Build history of the part. All positions in model axes, mm. A direction names the side the tool comes from. Give positions to 0.01 mm unless a question says otherwise; leave off trailing zeros. One line per item, written item: value.
```python
from build123d import *

# Parameters (mm, degrees)
F0_W     = 400
F0_H     = 400
F1_DEPTH = 30
F3_DEPTH = 20
F5_D     = 8.5


with BuildPart() as f1:
    # F0 (on Front) → F1 (new body)
    with BuildSketch(Plane.XZ):
        with Locations((200, 200)):
            Rectangle(F0_W, F0_H)
    extrude(amount=F1_DEPTH)

    # F2 (on face) → F3 (cut)
    with BuildSketch(Plane.XZ.offset(30)):
        with BuildLine():
            Line((7, 26), (0, 26))
            Line((0, 26), (0, 12))
            Line((0, 12), (7, 12))
            ThreePointArc((7, 12), (14, 19), (7, 26))
        make_face()
        with BuildLine():
            Line((393, 12), (400, 12))
            Line((400, 12), (400, 26))
            Line((400, 26), (393, 26))
            ThreePointArc((393, 26), (386, 19), (393, 12))
        make_face()
        with BuildLine():
            Line((400, 374), (400, 388))
            Line((400, 388), (393, 388))
            ThreePointArc((393, 388), (386, 381), (393, 374))
            Line((393, 374), (400, 374))
        make_face()
        with BuildLine():
            Line((0, 381), (0, 374))
            Line((0, 374), (7, 374))
            ThreePointArc((7, 374), (14, 381), (7, 388))
            Line((7, 388), (0, 388))
            Line((0, 388), (0, 381))
        make_face()
    extrude(amount=-F3_DEPTH, mode=Mode.SUBTRACT)

    # F5 (through all)
    with Locations(Plane.XZ.offset(10)):
        with Locations((7, 381), (393, 381), (393, 19), (7, 19)):
            Hole(F5_D / 2)


solid = f1.part
```
(1) Drill centre lines: line 1 (Z direction, x = 393, y = -5.5); line 2 (X direction, y = -2.25, z = 381); line 3 (X direction, y = -17.25, z = 382.5). Where is each one in solid material? Low to high.
Completed:
line 1: 0 to 14.75, 23.25 to 376.75, 385.25 to 400
line 2: 0 to 2.75, 11.25 to 388.75, 397.25 to 400
line 3: 13.84 to 386.16
(2) 3-axis set-ups, long thin cutter, end or side, ignore diameter. For faces 5 (the face through (396.132, -4.93, 383.872)), 6 (the face through (14, -20, 381)), 7 (the face through (398, -10, 381)): which of +Z, -Z, +X, -X, +Y, -Y reach the whole face in a straight line?
Completed:
face 5: +Y, -Y
face 6: -X, -Y
face 7: +X, -Y
(3) Pull direction X, two halves, no side cores. Call faces 1 (the face through (3.79, -10, 377.99)), 2 (the face through (7.553, -4.93, 385.214)), 3 (the face through (14, -20, 19)), 4 (the face through (397.246, -4.93, 19.187)): +X half, -X half, draft (parallel to the pull), parting line (faces both ways), or undercut.
Completed:
face 1: draft
face 2: undercut
face 3: -X half
face 4: undercut
(4) Pin check, flat tip, straight feed: P1, Ø4, axis at x = 395, z = 384.5, coming from the -Y side. Stop position of the tip, or through.
Completed:
P1: y = -10
